Part print with two shaded views. Sizes in mm from the minimum x, y, z corner. Round coordinates to 2 decimals unless told otherwise and drop trailing zeros. Order: outer loops, then holes, each group sorted by start corner. A loop starts at its lowest first (then second) coordinate and runs counter-clockwise, first axis right, second up. Notation, with made-up numbers: M 70.25,-29.75 L 114.25,-29.75 A28 ccw 114.25,-11.75 Z; hole C 25.25,75.5 d10. An arc over 180 degrees is marked long. Answer as a JSON object with one key per item and string values.
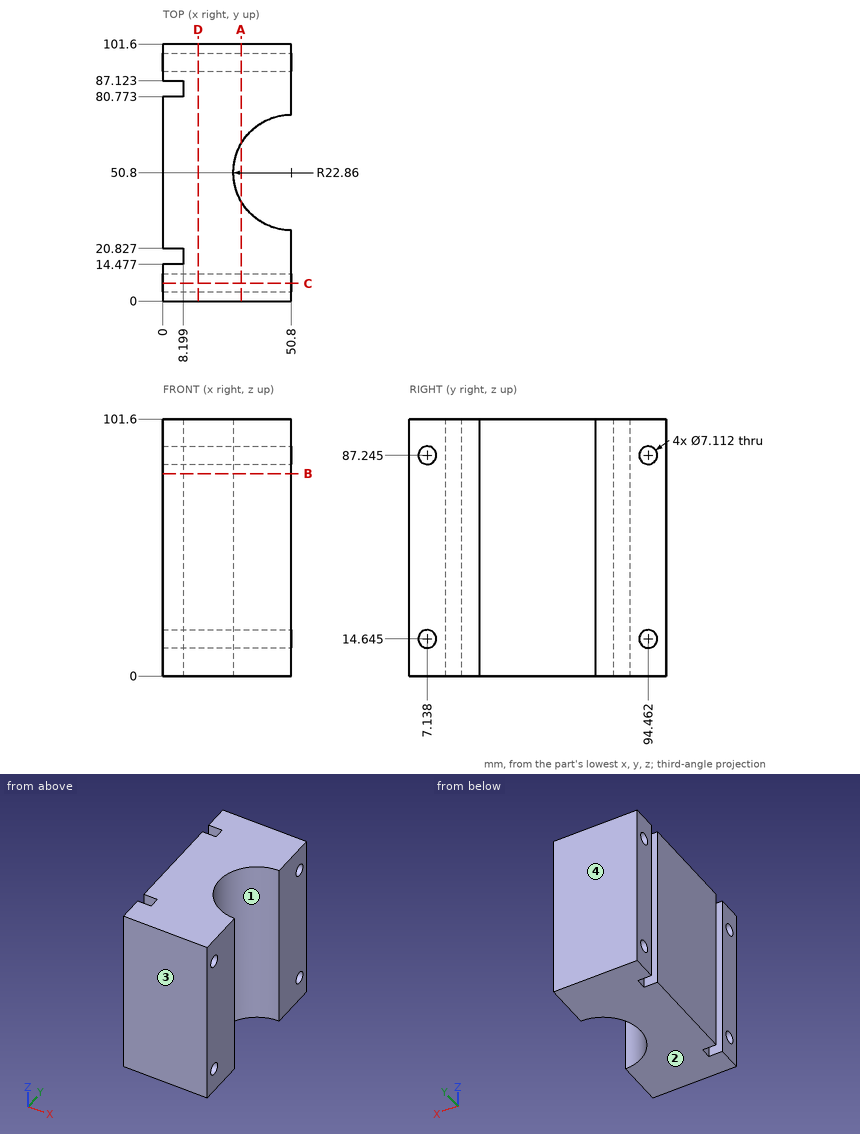
Item 1: Saw through at D-D on x = 14. List the corners of the cut face in (y, z) (1 decimal).
Worked answers:
{"outline": "M 0,0 L 101.6,0 L 101.6,101.6 L 0,101.6 Z; hole C 7.1,14.6 d7.1; hole C 7.1,87.2 d7.1; hole C 94.5,14.6 d7.1; hole C 94.5,87.2 d7.1"}
Item 2: Saw through at C-C on y = 7. List the corners of the cut face in (x, z), and give its area (3 significant figures).
Worked answers:
{"outline": "M 0,0 L 50.8,0 L 50.8,11.09 L 0,11.09 Z; M 0,18.2 L 50.8,18.2 L 50.8,83.69 L 0,83.69 Z; M 0,90.8 L 50.8,90.8 L 50.8,101.6 L 0,101.6 Z", "area": "4,440 mm2"}
Item 3: Saw through at A-A on x = 31. List the corners of the cut face in (y, z) (1 decimal).
Worked answers:
{"outline": "M 0,0 L 39.4,0 L 39.4,101.6 L 0,101.6 Z; M 62.2,0 L 101.6,0 L 101.6,101.6 L 62.2,101.6 Z; hole C 7.1,14.6 d7.1; hole C 7.1,87.2 d7.1; hole C 94.5,14.6 d7.1; hole C 94.5,87.2 d7.1"}
Item 4: Drop flat-ended pins along their axis: pin 1 Ø1.9 at (y, z) = (83, 32.5) entering from -X; pin 2 Ø4.5 at (y, z) = (7.14, 14.65) entering from +X; pin 3 Ø2 at (y, z) = (44, 90) entering from +X. Give the stop position or say it passes through.
Worked answers:
{"pin 1": "stops at x = 8.2", "pin 2": "passes through", "pin 3": "stops at x = 29.31"}
Item 5: Saw through at B-B on z = 80. List the corners of the cut face in (x, y), and give its area (3 significant figures).
Worked answers:
{"outline": "M 0,0 L 50.8,0 L 50.8,27.94 A22.86 cw 50.8,73.66 L 50.8,101.6 L 0,101.6 L 0,87.12 L 8.2,87.12 L 8.2,80.77 L 0,80.77 L 0,20.83 L 8.2,20.83 L 8.2,14.48 L 0,14.48 Z", "area": "4,240 mm2"}
Item 6: Two-plate mould, pull along Y, no slides. Class the marked faces 1, 2, 3 and 4: released by +Y, released by -Y, zero draft, split by the parting line, or undercut.
Worked answers:
{"face 1": "undercut", "face 2": "zero draft", "face 3": "released by -Y", "face 4": "released by +Y"}
Item 7: Wall check: line 1 along Y through (x, z) = (8, 46); line 2 along Y through (x, z) = (10, 87.5) (1 decimal); line 3 along Z through (x, y) = (39.5, 91.5). Give the ranges that are in metal, low to high. Write a range as [from, to].
Worked answers:
{"line 1": "y = [0, 14.48], [20.83, 80.77], [87.12, 101.6]", "line 2": "y = [0, 3.6], [10.7, 90.9], [98, 101.6]", "line 3": "z = [0, 12.68], [16.61, 85.28], [89.21, 101.6]"}
